from build123d import *

# Parameters (mm, degrees)
SKETCH_1_R                   = 3
EXTRUDE_1_DEPTH              = 19
SKETCH_2_W                   = 1
SKETCH_2_H                   = 10
CUT_EXTRUDE_2_DEPTH          = 9.25
HOLE_WIZARD_M3_1_D           = 2.5
HOLE_WIZARD_M3_1_DEPTH       = 7.5
HOLE_WIZARD_M3_1_CBORE_D     = 3
HOLE_WIZARD_M3_1_CBORE_DEPTH = 6
HOLE_WIZARD_M3_1_TIP         = 0.751075774
SKETCH_4_R                   = 1.5
EXTRUDE_3_DEPTH              = 6


with BuildPart() as part:
    # 草图1 → 拉伸1 (new body)
    with BuildSketch(Plane.XY):
        Circle(SKETCH_1_R)
    extrude(amount=EXTRUDE_1_DEPTH)

    # 草图2 → 拉伸2 (cut, symmetric)
    with BuildSketch(Plane(origin=(0, 0, 0), x_dir=(1, 0, 0), z_dir=(0, 1, 0))):
        with Locations((-2.5, -10)):
            Rectangle(SKETCH_2_W, SKETCH_2_H)
        with Locations((2.5, -10)):
            Rectangle(SKETCH_2_W, SKETCH_2_H)
    extrude(amount=CUT_EXTRUDE_2_DEPTH, both=True, mode=Mode.SUBTRACT)

    # M3 螺纹孔1
    with Locations(Plane(origin=(0, 0, 0), x_dir=(-1, 0, 0), z_dir=(0, 0, -1))):
        with Locations((0, 0)):
            CounterBoreHole(HOLE_WIZARD_M3_1_D / 2, HOLE_WIZARD_M3_1_CBORE_D / 2, HOLE_WIZARD_M3_1_CBORE_DEPTH, depth=HOLE_WIZARD_M3_1_DEPTH)
            with Locations((0, 0, -(HOLE_WIZARD_M3_1_DEPTH + HOLE_WIZARD_M3_1_TIP / 2))):  # 118° drill point
                Cone(0, HOLE_WIZARD_M3_1_D / 2, HOLE_WIZARD_M3_1_TIP, mode=Mode.SUBTRACT)

    # 草图4 → 拉伸3 (add)
    with BuildSketch(Plane.XY.offset(19)):
        with Locations(Location((0, 0, 0), (0, 0, 180))):
            Circle(SKETCH_4_R)
    extrude(amount=EXTRUDE_3_DEPTH)


solid = part.part
Model file for the job. Use its own axes, mm. A direction names the side the tool comes from. Give positions to 0.01 mm unless a question says otherwise; leave off trailing zeros. Order: outer loops, then holes, each group sorted by start corner. A loop starts at its lowest first (then second) coordinate and runs counter-clockwise, first axis right, second up. Notation, with made-up numbers: (19.25, 29) - (63.25, 29) arc R11 cw to (63.25, 47) - close; hole circle Ø10 at (42.5, 38.25). An arc over 180 degrees is marked (long way). Return JSON: item names as keys, results as strings.
1) Flat gauge pins, fed straight in: P1, Ø1.5, axis at y = -1.5, z = 16.5, coming from the -X side; P2, Ø0.5, axis at x = -2.5, y = 1, coming from the +Z side; P3, Ø3.5, axis at y = -1, z = 10, coming from the -X side. Where does each tip first touch, or does it go through?
Geometry says:
{"P1": "x = -2.9", "P2": "z = 19", "P3": "x = -2"}
2) Cut at D-D, the plane y = 1.75. Give the cut face in (x, z).
Geometry says:
{"outline": "(-2.44, 0) - (2.44, 0) - (2.44, 5) - (2, 5) - (2, 15) - (2.44, 15) - (2.44, 19) - (-2.44, 19) - (-2.44, 15) - (-2, 15) - (-2, 5) - (-2.44, 5) - close"}
3) Pull direction Z, two halves, no side cores. Call faces 1 (the flat face through (1.3, -1.3, 19)), 2 (the flat face through (2.4, 0, 15)), 3 (the cylindrical face through (1.5, 0.07, 2.96)): pulls with the +Z half, pulls with the -Z half, needs draft (parallel to the pull), parting line crosses it, or undercut.
Geometry says:
{"face 1": "pulls with the +Z half", "face 2": "undercut", "face 3": "needs draft"}
4) Cut at B-B, the plane z = 5.25. Give the cut face in (x, y).
Geometry says:
{"outline": "(-2, -2.24) arc R3 ccw to (2, -2.24) - (2, 2.24) arc R3 ccw to (-2, 2.24) - close; hole circle Ø3 at (0, 0)"}
5) Cut at A-A, the plane y = -1.8. Give the cut face in (x, z), plus the area to 3 significant figures.
Geometry says:
{"outline": "(-2.4, 0) - (2.4, 0) - (2.4, 5) - (2, 5) - (2, 15) - (2.4, 15) - (2.4, 19) - (-2.4, 19) - (-2.4, 15) - (-2, 15) - (-2, 5) - (-2.4, 5) - close", "area": "83.2 mm²"}
6) Probe line 1 (Y direction, x = 0, z = 6.75); line 2 (Z direction, x = -2.55, y = -1.1); line 3 (X direction, y = 0, z = 6.8). List the from-to ranges inside material, lowest first. Write a range as from..to.
Geometry says:
{"line 1": "-3..-1.25, 1.25..3", "line 2": "0..5, 15..19", "line 3": "-2..-1.25, 1.25..2"}
7) Cut at C-C, the plane z = 14.75. Give the cut face in (x, y), plus the area to 3 significant figures.
Geometry says:
{"outline": "(-2, -2.24) arc R3 ccw to (2, -2.24) - (2, 2.24) arc R3 ccw to (-2, 2.24) - close", "area": "22.1 mm²"}
8) 3-axis set-ups, long thin cutter, end or side, ignore diameter. For faces 4 (the cylindrical face through (-0.27, -1.22, 6.76)), 5 (the flat face through (-2, 0, 10)), 6 (the flat face through (2, 0, 10)), 7 (the cylindrical face through (1.384, -2.662, 9.367)), 8 (the cylindrical face through (-1.43, -0.45, 21.96)): which of +Z, -Z, +X, -X, +Y, -Y reach the whole face in a straight line?
Geometry says:
{"face 4": "-Z", "face 5": "-X, +Y, -Y", "face 6": "+X, +Y, -Y", "face 7": "+Z, -Z", "face 8": "+Z"}
